Read the model definition and answer for the solid it produces. Units are mm, in the model's axes. Face numbers are marked on the shaded views. Round coordinates to 2 decimals unless told otherwise and drop trailing zeros. Write each loop counter-clockwise with the first axis right and the second up, starting at its lowest first coordinate (ties: lowest second). Pieces come first, ordered by that corner, then holes. Notation, with made-up numbers: (7.25, -21) - (52.25, -21) arc R29 ccw to (52.25, 1) - close; hole circle Ø9 at (10, 25.5). An arc over 180 degrees is marked (long way). One line per item, written item: value. Start each with the question number.
(1) A cutting plane is placed at D-D, the plane y = -8. Determine the outline of the cut face in (x, z).
(2) A cutting plane is placed at C-C, the plane z = 2.25. Determine the outline of the cut face in (x, y).
(3) A cutting plane is placed at B-B, the plane x = -7. Determine the outline of the cut face in (y, z), plus the area to 3 significant figures.
(4) A cutting plane is placed at A-A, the plane y = 0. Determine the outline of the cut face in (x, z), plus the area to 3 significant figures.
(5) The mould has two halves that part along Y. Classify the marked faces 1, 2, 3 and 4: +Y half, -Y half, draft (parallel to the pull), parting line (faces both ways), or undercut.
(6) Flat-ended cylindrical pins translate along their axes: pin 1 Ø1.9 at (x, y) = (20, 0) entering from -Z; pin 2 Ø1 at (x, z) = (13, 3) entering from +Y; pin 3 Ø1 at (y, z) = (10.5, 2) entering from +X; pin 4 Ø1 at (y, z) = (10, 1.5) entering from +X. Find the tip coordinate at first contact, or state that the pin passes through.
(7) Find the intervals of material crossed by L1, parallel to Y at x = 8, z = 2.6; L2, parallel to X at y = 1, z = 1.6; L3, parallel to X at y = 3, z = 2.3, in increasing order.
from build123d import *

# Parameters (mm, degrees)
SKETCH_R  = 1.6
SKETCH_W  = 32
SKETCH_H  = 22
PAD_DEPTH = 3.2


with BuildPart() as part:
    # Sketch → Pad (new body)
    with BuildSketch(Plane.XY):
        with BuildLine():
            Line((-9.5, 17.5), (9.5, 17.5))
            ThreePointArc((23.5, 3.5), (19.399495, 13.399495), (9.5, 17.5))
            Line((23.5, 3.5), (23.5, -3.5))
            ThreePointArc((9.5, -17.5), (19.399495, -13.399495), (23.5, -3.5))
            Line((9.5, -17.5), (-9.5, -17.5))
            ThreePointArc((-23.5, -3.5), (-19.399495, -13.399495), (-9.5, -17.5))
            Line((-23.5, -3.5), (-23.5, 3.5))
            ThreePointArc((-9.5, 17.5), (-19.399495, 13.399495), (-23.5, 3.5))
        make_face()
        with Locations((-20, 0)):
            Circle(SKETCH_R, mode=Mode.SUBTRACT)
        with Locations((20, 0)):
            Circle(SKETCH_R, mode=Mode.SUBTRACT)
        Rectangle(SKETCH_W, SKETCH_H, mode=Mode.SUBTRACT)
    extrude(amount=PAD_DEPTH)


solid = part.part
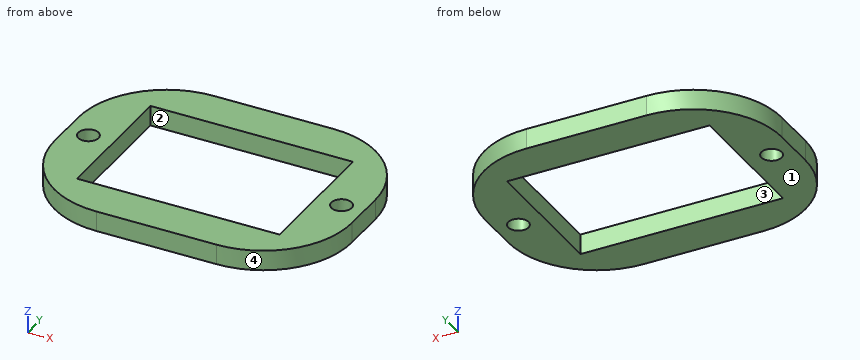
Here are the results:
1. outline: (-22.76, 0) - (-16, 0) - (-16, 3.2) - (-22.76, 3.2) - close; (16, 0) - (22.76, 0) - (22.76, 3.2) - (16, 3.2) - close
2. outline: (-23.5, -3.5) arc R14 ccw to (-9.5, -17.5) - (9.5, -17.5) arc R14 ccw to (23.5, -3.5) - (23.5, 3.5) arc R14 ccw to (9.5, 17.5) - (-9.5, 17.5) arc R14 ccw to (-23.5, 3.5) - close; hole circle Ø3.2 at (-20, 0); hole (-16, -11) - (16, -11) - (16, 11) - (-16, 11) - close; hole circle Ø3.2 at (20, 0)
3. outline: (-17.5, 0) - (-11, 0) - (-11, 3.2) - (-17.5, 3.2) - close; (11, 0) - (17.5, 0) - (17.5, 3.2) - (11, 3.2) - close
3. area: 41.6 mm²
4. outline: (-23.5, 0) - (-21.6, 0) - (-21.6, 3.2) - (-23.5, 3.2) - close; (-18.4, 0) - (-16, 0) - (-16, 3.2) - (-18.4, 3.2) - close; (16, 0) - (18.4, 0) - (18.4, 3.2) - (16, 3.2) - close; (21.6, 0) - (23.5, 0) - (23.5, 3.2) - (21.6, 3.2) - close
4. area: 27.5 mm²
5. face 1: draft
5. face 2: undercut
5. face 3: undercut
5. face 4: -Y half
6. pin 1: through
6. pin 2: y = 17.17
6. pin 3: x = 21.9
6. pin 4: x = 22.15
7. L1: -17.5 to -11, 11 to 17.5
7. L2: -23.5 to -21.25, -18.75 to -16, 16 to 18.75, 21.25 to 23.5
7. L3: -23.5 to -16, 16 to 23.5
